```python
from build123d import *

# Parameters (mm, degrees)
SKETCH2_R                = 19
SKETCH2_R_2              = 15
BOSS_EXTRUDE1_DEPTH      = 0.5
SKETCH3_R                = 20
BOSS_EXTRUDE2_DEPTH      = 9.5
CUT_EXTRUDE2_START       = -6
CUT_EXTRUDE2_DEPTH       = 6
M3_CLEARANCE_HOLE1_D     = 3.4
M3_CLEARANCE_HOLE1_DEPTH = 5
M3_CLEARANCE_HOLE1_TIP   = 1.021463052


with BuildPart() as part:
    # Sketch2 → Boss-Extrude1 (new body)
    with BuildSketch(Plane(origin=(0, 0, 0), x_dir=(0, 1, 0), z_dir=(0, 0, 1))):
        with Locations(Location((0, 0, 0), (0, 0, 270))):
            Circle(SKETCH2_R)
        with Locations(Location((0, 0, 0), (0, 0, 270))):
            Circle(SKETCH2_R_2, mode=Mode.SUBTRACT)
    extrude(amount=-BOSS_EXTRUDE1_DEPTH)

    # Sketch3 → Boss-Extrude2 (add)
    with BuildSketch(Plane(origin=(0, 0, -0.5), x_dir=(1, 0, 0), z_dir=(0, 0, -1))):
        with Locations(Location((0, 0, 0), (0, 0, 180))):
            Circle(SKETCH3_R)
    extrude(amount=BOSS_EXTRUDE2_DEPTH)

    # Sketch4 → Cut-Extrude2 (cut)
    with BuildSketch(Plane(origin=(0, 0, -10), x_dir=(1, 0, 0), z_dir=(0, 0, -1)).offset(CUT_EXTRUDE2_START)):
        with BuildLine():
            Line((-5, -17.5), (-5, -19.364916731))
            ThreePointArc((-5, -19.364916731), (0, -20), (5, -19.364916731))
            Line((5, -19.364916731), (5, -17.5))
            ThreePointArc((5, -17.5), (4.267766953, -15.732233047), (2.5, -15))
            Line((2.5, -15), (-2.5, -15))
            ThreePointArc((-2.5, -15), (-4.267766953, -15.732233047), (-5, -17.5))
        make_face()
    extrude(amount=CUT_EXTRUDE2_DEPTH, mode=Mode.SUBTRACT)

    # M3 Clearance Hole1
    with Locations(Plane(origin=(0, 0, -10), x_dir=(1, 0, 0), z_dir=(0, 0, -1))):
        with Locations((-8.838834765, -8.838834765), (8.838834765, -8.838834765), (8.838834765, 8.838834765), (-8.838834765, 8.838834765)):
            Hole(M3_CLEARANCE_HOLE1_D / 2, depth=M3_CLEARANCE_HOLE1_DEPTH)
            with Locations((0, 0, -(M3_CLEARANCE_HOLE1_DEPTH + M3_CLEARANCE_HOLE1_TIP / 2))):  # 118° drill point
                Cone(0, M3_CLEARANCE_HOLE1_D / 2, M3_CLEARANCE_HOLE1_TIP, mode=Mode.SUBTRACT)


solid = part.part
```
Check sheet for the modelled part. Datum: model origin and axes. Units: mm. A direction names the side the tool comes from. Give positions to 0.01 mm unless a question says otherwise; leave off trailing zeros. Write each loop counter-clockwise with the first axis right and the second up, starting at its lowest first coordinate (ties: lowest second). Pieces come first, ordered by that corner, then holes.
Item 1: Cross-section at A-A (y = 0). Enter the section's corners in (x, z), and give its area (3 significant figures).
Item 2: Scan lines: L1, parallel to Y at x = 0, z = -0.3; L2, parallel to Y at x = 8.5, z = -8; L3, parallel to X at y = -9.5, z = -6.5 (3 decimals). Record each from-to range of solid material in increasing order.
Item 3: Gauge pin test, flat ends, axial feed: pin 1 (5 mm diameter, centred on y = -11.5, z = -3.5, fed in from +X); pin 2 (6 mm diameter, centred on x = 3.5, z = -4.5, fed in from -Y); pin 3 (0.9 mm diameter, centred on y = 18.5, z = -8, fed in from +X); pin 4 (8 mm diameter, centred on x = 15.5, y = 3, fed in from +Z). Record the tip position at first contact, or that the pin passes through.
Item 4: Cross-section at B-B (x = 0). Enter the section's corners in (y, z).
Item 5: Access from +Z, -Z, +X, -X, +Y, -Y to the whole of each face (thin tool, end or side, straight path). Record for faces 4 (the face through (-8.47, -7.18, -7.46)), 5 (the face through (4.287, 15.752, -6.958)), 6 (the face through (0, 0, -0.5)), 7 (the face through (4.336, -19.524, -5.184)), 8 (the face through (0, 0, -10)).
Item 6: Cross-section at C-C (z = -7). Enter the section's corners in (x, y).
Item 7: Draft check along Y on faces 1 (the face through (-8.47, 10.5, -7.46)), 2 (the face through (14, 6, 0)), 3 (the face through (0, 15, -7)). Enter one of: released by +Y, released by -Y, zero draft, split by the parting line, or undercut.
Item 8: Cross-section at D-D (z = -1.25). Enter the section's corners in (x, y), and give its area (3 significant figures).
Report:
1. outline: (-20, -10) - (20, -10) - (20, -0.5) - (19, -0.5) - (19, 0) - (15, 0) - (15, -0.5) - (-15, -0.5) - (-15, 0) - (-19, 0) - (-19, -0.5) - (-20, -0.5) - close
1. area: 384 mm2
2. L1: y = -19 to -15, 15 to 19
2. L2: y = -18.1 to -10.5, -7.17 to 7.17, 10.5 to 18.1
2. L3: x = -17.6 to -10.405, -7.273 to 7.273, 10.405 to 17.6
3. pin 1: stops at x = 17.86
3. pin 2: stops at y = -19.99
3. pin 3: stops at x = 8.61
3. pin 4: stops at z = 0
4. outline: (-20, -10) - (15, -10) - (15, -4) - (20, -4) - (20, -0.5) - (19, -0.5) - (19, 0) - (15, 0) - (15, -0.5) - (-15, -0.5) - (-15, 0) - (-19, 0) - (-19, -0.5) - (-20, -0.5) - close
5. face 4: -Z
5. face 5: -Z, +Y
5. face 6: +Z
5. face 7: +Z, -Z
5. face 8: -Z, +X, -X, +Y, -Y
6. outline: (-5, 17.5) - (-5, 19.36) arc R20 ccw (long way) to (5, 19.36) - (5, 17.5) arc R2.5 cw to (2.5, 15) - (-2.5, 15) arc R2.5 cw to start; hole circle Ø3.4 at (-8.84, -8.84); hole circle Ø3.4 at (-8.84, 8.84); hole circle Ø3.4 at (8.84, -8.84); hole circle Ø3.4 at (8.84, 8.84)
7. face 1: undercut
7. face 2: zero draft
7. face 3: released by +Y
8. outline: circle Ø40 at (0, 0)
8. area: 1,260 mm2
